from build123d import *

# Parameters (mm, degrees)
SKETCH_4_R           = 2.0000000000000924
SKETCH_4_R_2         = 2.5
EXTRUDE_1_DEPTH      = 5
EXTRUDE_2_DEPTH      = 7
EXTRUDE_2_DEPTH_BACK = 5
FILLET_3_R           = 1.5
FILLET_4_R           = 1.5
SKETCH_6_R           = 3.0000000000000897
SKETCH_6_R_2         = 2.0000000000000884
EXTRUDE_3_DEPTH      = 0.5


with BuildPart() as part:
    # 草图4 → 凸台-拉伸1 (new body)
    with BuildSketch(Plane.XY):
        with BuildLine():
            Line((4.306700056173786, 1.3047354621350271), (14.109660641900325, -5.571834508606824))
            ThreePointArc((14.109660641900325, -5.571834508606824), (17.74630975952625, -10.35823275650958), (11.807053976651485, -11.285630048852315))
            Line((11.807053976651485, -11.285630048852315), (1.6735833284293933, -4.177214244302438))
            ThreePointArc((1.6735833284293933, -4.177214244302438), (-4.056339542742652, 1.948360724810045), (4.306700056173786, 1.3047354621350271))
        make_face()
        with Locations((14.500000000000004, -9.05)):
            Circle(SKETCH_4_R, mode=Mode.SUBTRACT)
        Circle(SKETCH_4_R_2, mode=Mode.SUBTRACT)
    extrude(amount=EXTRUDE_1_DEPTH)

    # 草图5 → 凸台-拉伸2 (add, two sides: drawn at the far end of the back side and taken through both)
    with BuildSketch(Plane(origin=(0, 0, 0), x_dir=(-1, 0, 0), z_dir=(0, 0, -1)).offset(-EXTRUDE_2_DEPTH_BACK)):
        Polygon((-0.6347261790104263, -3.4484778778636556), (-7.184027973017892, -8.042674870920285), (-10.629675717810366, -3.130698525414685), (-4.080373923802897, 1.463498467641941), align=None)
    extrude(amount=EXTRUDE_2_DEPTH + EXTRUDE_2_DEPTH_BACK)

    # 圆角3
    fillet_3_edges = [part.edges().sort_by_distance(p)[0] for p in [
        (8.90685184541413, -5.586686698167485, 0),
        (4.306700056173785, 1.3047354621350273, 2.5),
    ]]
    fillet(fillet_3_edges, radius=FILLET_3_R)

    # 圆角4
    fillet_4_edges = [part.edges().sort_by_distance(p)[0] for p in [
        (11.807053976651485, -11.285630048852315, 2.5),
        (1.6735833284293933, -4.177214244302439, 2.5),
    ]]
    fillet(fillet_4_edges, radius=FILLET_4_R)

    # 草图6 → 凸台-拉伸3 (add)
    with BuildSketch(Plane.XY.offset(5)):
        with Locations((14.500000000000004, -9.05)):
            Circle(SKETCH_6_R)
        with Locations((14.500000000000004, -9.05)):
            Circle(SKETCH_6_R_2, mode=Mode.SUBTRACT)
    extrude(amount=EXTRUDE_3_DEPTH)


solid = part.part
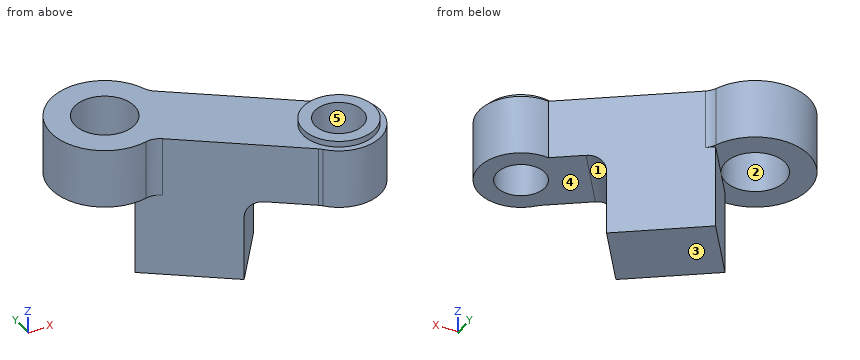
Design review of the part built by this model. Coordinates are the model's own, in mm. Face numbers are marked on the shaded views. A direction names the side the tool comes from. Coordinates: 2 decimals unless noted, no trailing zeros. Order: outer loops, then holes, each group sorted by start corner. A loop starts at its lowest first (then second) coordinate and runs counter-clockwise, first axis right, second up.
Item 1: Take a section at A-A, the plane x = 14.5. Write out the cut boundary in (y, z).
Item 2: For pin 1 Ø4.5 at (x, y) = (1, -1) entering from -Z; pin 2 Ø7 at (x, y) = (15, -6.5) entering from -Z; pin 3 Ø3.5 at (x, y) = (14.5, -9.05) entering from +Z; pin 4 Ø2 at (x, z) = (8, -1) entering from -Y, all flat-tipped, find the tip position at first contact; note any pin that passes through.
Item 3: For the marked faces 4 and 5, list the 3-axis set-ups (+Z, -Z, +X, -X, +Y, -Y) from which the entire face can be reached by the end or side of a thin tool; tool diameter is ignored.
Item 4: Take a section at B-B, the plane y = 0. Write out the cut boundary in (x, z).
Item 5: Take a section at D-D, the plane x = -1.25. Write out the cut boundary in (y, z), then the cut area to 3 significant figures.
Item 6: Take a section at C-C, the plane z = 3.25. Write out the cut boundary in (x, y).
Item 7: The part is to be moulded in two halves that separate along X. For the marked faces 1, 2 and 3, say which applies: pulls with the +X half, pulls with the -X half, needs draft (parallel to the pull), parting line crosses it, or undercut.
Item 8: For line 1 (Y direction, x = 0, z = 2.55); line 2 (Z direction, x = 4.5, y = -0.5); line 3 (Z direction, x = 10, y = -8.25), list the stretches that pass through material, from the lowest coordinate up.
The answers:
1. outline: (-12.55, 0) - (-11.05, 0) - (-11.05, 5.5) - (-12.05, 5.5) - (-12.05, 5) - (-12.55, 5) - close; (-7.05, 0) - (-5.55, 0) - (-5.55, 5) - (-6.05, 5) - (-6.05, 5.5) - (-7.05, 5.5) - close
2. pin 1: stops at z = -7
2. pin 2: stops at z = 0
2. pin 3: passes through
2. pin 4: stops at y = -8.76
3. face 4: -Z, +X, -Y
3. face 5: +Z, -Z
4. outline: (-4.5, 0) - (-2.5, 0) - (-2.5, 5) - (-4.5, 5) - close; (2.5, 0) - (3.05, 0) - (3.05, -7) - (6.17, -7) - (6.17, 5) - (2.5, 5) - close
5. outline: (-4.32, 0) - (-2.17, 0) - (-2.17, 5) - (-4.32, 5) - close; (2.17, 0) - (4.32, 0) - (4.32, 5) - (2.17, 5) - close
5. area: 21.6 mm2
6. outline: (1.06, -4.37) arc R1.5 cw to (2.28, -4.6) - (11.66, -11.18) arc R1.5 cw to (11.91, -11.4) arc R3.5 ccw (long way) to (14.11, -5.57) - (4.7, 1.03) arc R1.5 cw to (4.17, 1.69) arc R4.5 ccw (long way) to start; hole circle Ø5 at (0, 0); hole circle Ø4 at (14.5, -9.05)
7. face 1: pulls with the +X half
7. face 2: undercut
7. face 3: needs draft
8. line 1: y = -4.5 to -2.5, 2.5 to 4.5
8. line 2: z = -7 to 5
8. line 3: z = 0 to 5
